Part model, mm, in its own coordinate system. Face numbers are marked on the shaded views. A direction names the side the tool comes from. Give positions to 0.01 mm unless a question says otherwise; leave off trailing zeros. Order: outer loops, then holes, each group sorted by start corner. A loop starts at its lowest first (then second) coordinate and runs counter-clockwise, first axis right, second up. Notation, with made-up numbers: (68, -6.5) - (80, -6.5) arc R27 ccw to (80, 19.5) - close; hole circle Ø8 at (73, 39.5). An arc over 180 degrees is marked (long way). One line per item, written item: value.
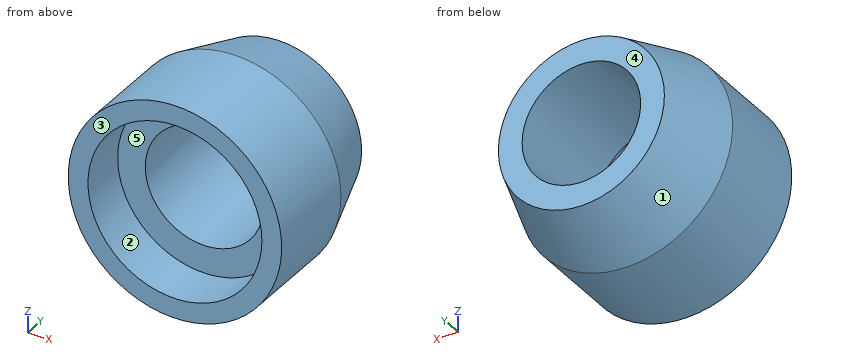
Autodesk Inventor part; units mm, degrees
ref_plane "YZ Plane" through (0, 0, 0) normal (1, 0, 0) x (0, 1, 0)
ref_plane "XZ Plane" through (0, 0, 0) normal (0, 1, 0) x (-1, 0, 0)
ref_plane "XY Plane" through (0, 0, 0) normal (0, 0, 1) x (1, 0, 0)
ref_plane "作業平面1" through (-45.0235, 27.1998, 9.5426) normal (0, 0, 1) x (1, 0, 0)
sketch "スケッチ2" plane through (0, 0, 0) normal (0, 0, 1) x (1, 0, 0)
  line L0 (7.5, 21) -> (7.5, 6)
  line L1 (7.5, 6) -> (11, 6)
  line L2 (11, 6) -> (11, 0)
  line L3 (11, 0) -> (13.5, 0)
  line L4 (13.5, 0) -> (13.5, 12)
  line L5 (-2.7, 0) -> (16.2, 0)
  line L6 (0, -4.2) -> (0, 25.2)
  line L7 (7.5, 21) -> (10.5, 21)
  line L8 (10.5, 21) -> (13.5, 12)
  point P0 (0, 0)
  point P1 (11, 3)
  dimension "d5" = 11
  dimension "d6" = 6
  dimension "d8" = 7.5
  dimension "d9" = 2.5
  dimension "d10" = 12
  dimension "d11" = 15
  dimension "d13" = 3
revolve "回転1" add sketch "スケッチ2" angle 360 about axis through (0, -10, 0) along (0, 1, 0)
properties part number "LimitedView_Parts"
1) Slice it at D-D on y = 15.5. Write the cut outline in (x, z).
Answer:
outline: circle Ø24.67 at (0, 0); hole circle Ø15 at (0, 0)
2) Slice it at A-A on x = 0. Write the cut outline in (y, z).
Answer:
outline: (0, -13.5) - (12, -13.5) - (21, -10.5) - (21, -7.5) - (6, -7.5) - (6, -11) - (0, -11) - close; (0, 11) - (6, 11) - (6, 7.5) - (21, 7.5) - (21, 10.5) - (12, 13.5) - (0, 13.5) - close
3) Which spindle directions (+Z, -Z, +X, -X, +Y, -Y) get a long thin tool onto all of the face, cutting with end or side? Do the marked faces 4 and 5. Say none if no direction does.
Answer:
face 4: +Z, -Z, +X, -X, +Y
face 5: -Y
4) Drop flat-ended pins along their axis: P1, Ø11, axis at x = -5, z = 0.5, coming from the -Y side; P2, Ø1.5, axis at x = -1.5, y = 6.5, coming from the -Z side; P3, Ø8, axis at y = 14.5, z = -8.5, coming from the -X side. Give the stop position or say it passes through.
Answer:
P1: stops at y = 6
P2: stops at z = -13.48
P3: stops at x = -12.38
5) Wall check: line 1 along Z through (x, y) = (0, 11.25); line 2 along Z through (x, y) = (0, 1.9). Give the ranges that are in metal, low to high. Write a range as [from, to].
Answer:
line 1: z = [-13.5, -7.5], [7.5, 13.5]
line 2: z = [-13.5, -11], [11, 13.5]
6) Slice it at C-C on y = 9. Write the cut outline in (x, z).
Answer:
outline: circle Ø27 at (0, 0); hole circle Ø15 at (0, 0)
7) Two-plate mould, pull along Z, no slides. Class the marked faces 1, 2 and 3: pulls with the +Z half, pulls with the -Z half, needs draft (parallel to the pull), parting line crosses it, or undercut.
Answer:
face 1: parting line crosses it
face 2: undercut
face 3: needs draft
8) Slice it at B-B on z = 0. Write the cut outline in (x, y).
Answer:
outline: (-13.5, 0) - (-11, 0) - (-11, 6) - (-7.5, 6) - (-7.5, 21) - (-10.5, 21) - (-13.5, 12) - close; (7.5, 6) - (11, 6) - (11, 0) - (13.5, 0) - (13.5, 12) - (10.5, 21) - (7.5, 21) - close
